```python
from build123d import *

# Parameters (mm, degrees)
BOSS_EXTRUDE1_DEPTH = 2.921
CUT_EXTRUDE1_DEPTH  = 209.202762766


with BuildPart() as part:
    # Sketch1 → Boss-Extrude1 (new body)
    with BuildSketch(Plane(origin=(0, 0, 0), x_dir=(1, 0, 0), z_dir=(0, 1, 0))):
        Polygon((147.207095926, 39.444022474), (107.763073453, 107.763073453), (39.444022474, 147.207095926), (-39.444022474, 147.207095926), (-107.763073453, 107.763073453), (-147.207095926, 39.444022474), (-147.207095926, -39.444022474), (-107.763073453, -107.763073453), (-39.444022474, -147.207095926), (39.444022474, -147.207095926), (107.763073453, -107.763073453), (147.207095926, -39.444022474), align=None)
    extrude(amount=-BOSS_EXTRUDE1_DEPTH)

    # Sketch3 → Cut-Extrude1 (cut, through all)
    with BuildSketch(Plane(origin=(0, 0, 0), x_dir=(1, 0, 0), z_dir=(0, 1, 0))):
        Polygon((-98.138063951, 26.296014982), (-71.842048969, 71.842048969), (-26.296014982, 98.138063951), (26.296014982, 98.138063951), (71.842048969, 71.842048969), (98.138063951, 26.296014982), (98.138063951, -26.296014982), (71.842048969, -71.842048969), (26.296014982, -98.138063951), (-26.296014982, -98.138063951), (-71.842048969, -71.842048969), (-98.138063951, -26.296014982), align=None)
    extrude(amount=-CUT_EXTRUDE1_DEPTH, mode=Mode.SUBTRACT)


solid = part.part
```
Geometry check sheet. Reference: the model listing, model coordinates, mm. A direction names the side the tool comes from. Coordinates: 2 decimals unless noted, no trailing zeros. Write each loop counter-clockwise with the first axis right and the second up, starting at its lowest first coordinate (ties: lowest second). Pieces come first, ordered by that corner, then holes. Notation, with made-up numbers: (81, 85.5) -> (134, 85.5) arc R13 cw to (134, 93.5) -> close; hole circle Ø7 at (56, -37). An arc over 180 degrees is marked (long way). Use CSV: the item, a comma, the result in double quotes. Start each with the question number.
Item 1: Mould release check, pull along X, two halves, no side actions. Record for faces 3 (the flat face through (-127.2, -1.4, -74.1)), 4 (the flat face through (127.76, -1.44, -73.13)), 5 (the flat face through (-48.75, -1.44, 85.174)): released by +X, released by -X, zero draft, split by the parting line, or undercut.
Item 2: Thickness scan on line 1 (Z direction, x = -13.5, y = -0.25); line 2 (Z direction, x = 128.5, y = -1.25). Record the ranges inside material, lowest first.
Item 3: Cross-section at D-D, the plane x = -124.5. Record the cut outline in (y, z), plus the area to 3 significant figures.
Item 4: Cross-section at A-A, the plane y = -2.3. Record the cut outline in (x, z).
Item 5: Depth check by flat-ended pin: pin 1 Ø5 at (x, z) = (-108, -23) entering from +Y. Enter the tip coordinate at first touch or a pass-through.
Item 6: Cross-section at C-C, the plane z = -86. Record the cut outline in (x, y), plus the area to 3 significant figures.
Item 7: Set-up check for faces 1 (the flat face through (48.75, -1.44, -85.174)), 2 (the flat face through (-127.76, -1.44, 73.13)): record each of +Z, -Z, +X, -X, +Y, -Y from which the full face is reachable in a straight line by a thin tool's end or side.
Item 8: Cross-section at B-B, the plane x = -65.5. Record the cut outline in (y, z).
Answers:
1,face 3,"released by -X"
1,face 4,"released by +X"
1,face 5,"undercut"
2,line 1,"-147.21 to -98.14, 98.14 to 147.21"
2,line 2,"-71.85 to 71.85"
3,outline,"(-2.92, -78.77) -> (0, -78.77) -> (0, 78.77) -> (-2.92, 78.77) -> close"
3,area,"460 mm^2"
4,outline,"(-147.21, -39.44) -> (-107.76, -107.76) -> (-39.44, -147.21) -> (39.44, -147.21) -> (107.76, -107.76) -> (147.21, -39.44) -> (147.21, 39.44) -> (107.76, 107.76) -> (39.44, 147.21) -> (-39.44, 147.21) -> (-107.76, 107.76) -> (-147.21, 39.44) -> close; hole (-98.14, -26.3) -> (-71.84, -71.84) -> (-26.3, -98.14) -> (26.3, -98.14) -> (71.84, -71.84) -> (98.14, -26.3) -> (98.14, 26.3) -> (71.84, 71.84) -> (26.3, 98.14) -> (-26.3, 98.14) -> (-71.84, 71.84) -> (-98.14, 26.3) -> close"
5,pin 1,"y = 0"
6,outline,"(-120.33, -2.92) -> (-47.32, -2.92) -> (-47.32, 0) -> (-120.33, 0) -> close; (47.32, -2.92) -> (120.33, -2.92) -> (120.33, 0) -> (47.32, 0) -> close"
6,area,"427 mm^2"
7,face 1,"+Y, -Y"
7,face 2,"+Z, -X, +Y, -Y"
8,outline,"(-2.92, -132.16) -> (0, -132.16) -> (0, -75.5) -> (-2.92, -75.5) -> close; (-2.92, 75.5) -> (0, 75.5) -> (0, 132.16) -> (-2.92, 132.16) -> close"
